```python
from build123d import *

# Parameters (mm, degrees)
SKETCH1_W = 2.032
SKETCH1_H = 104.0892


with BuildPart() as part:
    # Sketch1 → Revolve1 (revolve)
    with BuildSketch(Plane(origin=(0, 0, 0), x_dir=(1, 0, 0), z_dir=(0, 1, 0))):
        with BuildLine():
            Line((8.4963, 64.4906), (5.715, 157.4546))
            ThreePointArc((5.715, 157.4546), (4.041115254, 161.495715254), (0, 163.1696))
            Line((0, 163.1696), (0, 52.0446))
            Line((0, 52.0446), (22.9743, 52.0446))
            Line((22.9743, 52.0446), (25.0063, 52.0446))
            Line((25.0063, 52.0446), (37.7063, 58.3946))
            Line((37.7063, 58.3946), (14.861271728, 58.330519522))
            ThreePointArc((14.861271728, 58.330519522), (10.4273746, 60.117525142), (8.4963, 64.4906))
        make_face()
        with Locations((23.9903, 0)):
            Rectangle(SKETCH1_W, SKETCH1_H)
    revolve(axis=Axis((0, 0, 52.0446), (0, 0, -1)))


solid = part.part
```
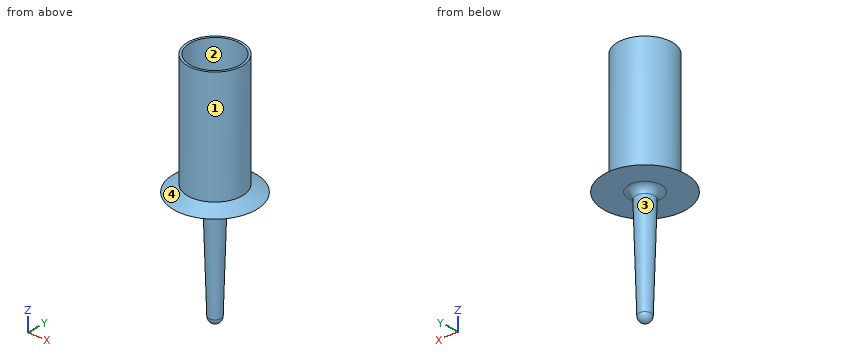
Source: CAD feature listing. Evaluate the final solid. Frame: model axes, mm. Face numbers are marked on the shaded views. A direction names the side the tool comes from. Round coordinates to 2 decimals unless told otherwise and drop trailing zeros. Loops run counter-clockwise (first coordinate to the right, second up) from the corner with the lowest first, then second, coordinate; pieces in that order, holes last. Notation, with made-up numbers: M 39,82.5 L 69,82.5 A25 ccw 69,102.5 Z; hole C 1,28 d1. An arc over 180 degrees is marked long. Use a Markdown table: item, result. Add a question column.
1. Reachability of the marked faces 3 and 4 from +Z, -Z, +X, -X, +Y, -Y: full face, straight path, thin tool, end or side. Return the list, or none.
2. Mould query, pull axis X, two halves, no side actions, for the marked faces 1 and 2. Classes: pulls with the +X half, pulls with the -X half, needs draft (parallel to the pull), parting line crosses it, or undercut.
3. Contact query for flat-ended pins moving along their axis: P1, Ø2, axis at y = -14.5, z = -24, coming from the -X side; P2, Ø8, axis at y = -27, z = -14.5, coming from the -X side; P3, Ø6, axis at x = -4.5, z = 30, coming from the -Y side. Output: stop coordinate, or through.
4. Line query: line 1 (X direction, y = 0, z = 20); line 2 (X direction, y = 12, z = 27). Output: solid intervals per line, ascending.
5. Section query D-D on z = -54. Return the cut outline in (x, y).
6. Section query C-C on z = -26. Return the cut outline in (x, y), then the cut area to 3 significant figures.
Reported:
| question | item | result |
|---|---|---|
| 1 | face 3 | -Z |
| 1 | face 4 | +Z |
| 2 | face 1 | parting line crosses it |
| 2 | face 2 | undercut |
| 3 | P1 | stops at x = -21.05 |
| 3 | P2 | stops at x = -9.81 |
| 3 | P3 | stops at y = -24.96 |
| 4 | line 1 | x = -25.01 to -22.97, 22.97 to 25.01 |
| 4 | line 2 | x = -21.94 to -19.59, 19.59 to 21.94 |
| 5 | outline | C 0,0 d57.83 |
| 6 | outline | C 0,0 d50.01; hole C 0,0 d45.95 |
| 6 | area | 306 mm² |
